Build history of the part. All positions in model axes, mm. Round coordinates to 2 decimals unless told otherwise and drop trailing zeros. Write each loop counter-clockwise with the first axis right and the second up, starting at its lowest first coordinate (ties: lowest second). Pieces come first, ordered by that corner, then holes.
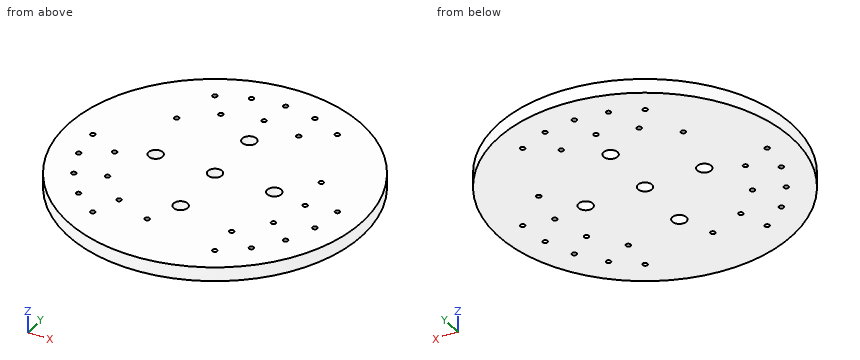
from build123d import *

# Parameters (mm, degrees)
SKETCH_R                          = 125.5
SKETCH_R_2                        = 6
PAD_DEPTH                         = 12
SKETCH001_R                       = 6
POCKET_DEPTH                      = 722.341763
POLARPATTERN_COUNT                = 4
SKETCH003_R                       = 2
POCKET001_DEPTH                   = 722.341763
SKETCH004_R                       = 2
POCKET002_DEPTH                   = 722.341763
SKETCH004_POLARPATTERN002_2_R     = 2
POCKET002_POLARPATTERN002_2_DEPTH = 722.341763
SKETCH004_POLARPATTERN002_3_R     = 2
POCKET002_POLARPATTERN002_3_DEPTH = 722.341763
SKETCH004_POLARPATTERN002_4_R     = 2
POCKET002_POLARPATTERN002_4_DEPTH = 722.341763
SKETCH004_POLARPATTERN002_5_R     = 2
POCKET002_POLARPATTERN002_5_DEPTH = 722.341763
POLARPATTERN003_COUNT             = 3
SKETCH003_POLARPATTERN004_2_R     = 2
POCKET001_POLARPATTERN004_2_DEPTH = 722.341763
SKETCH003_POLARPATTERN004_3_R     = 2
POCKET001_POLARPATTERN004_3_DEPTH = 722.341763
SKETCH003_POLARPATTERN004_4_R     = 2
POCKET001_POLARPATTERN004_4_DEPTH = 722.341763
POLARPATTERN005_COUNT             = 3


with BuildPart() as part:
    # Sketch → Pad (new body)
    with BuildSketch(Plane.XY):
        Circle(SKETCH_R)
        Circle(SKETCH_R_2, mode=Mode.SUBTRACT)
    extrude(amount=PAD_DEPTH)

    # Sketch001 → Pocket (cut, through all)
    with BuildSketch(Plane(origin=(0, 0, 0), x_dir=(-1, 0, 0), z_dir=(0, 0, -1))):
        with Locations((0, 50)):
            Circle(SKETCH001_R)
    pocket = extrude(amount=-POCKET_DEPTH, mode=Mode.SUBTRACT)

    # PolarPattern: Pocket ×4 about axis
    polarpattern_axis = Axis((0, 0, 0), (0, 0, -1))
    for i in range(1, POLARPATTERN_COUNT):
        add(pocket.rotate(polarpattern_axis, i * 360 / POLARPATTERN_COUNT), mode=Mode.SUBTRACT)

    # Sketch003 → Pocket001 (cut, through all)
    with BuildSketch(Plane.XY.offset(12)):
        with Locations((28.131884, 73.286063)):
            Circle(SKETCH003_R)
    pocket001 = extrude(amount=-POCKET001_DEPTH, mode=Mode.SUBTRACT)

    # Sketch004 → Pocket002 (cut, through all)
    with BuildSketch(Plane.XY.offset(12)):
        with Locations((51.453015, 89.227727)):
            Circle(SKETCH004_R)
    pocket002 = extrude(amount=-POCKET002_DEPTH, mode=Mode.SUBTRACT)

    # Sketch004 PolarPattern002 2 → Pocket002 PolarPattern002 2 (cut, through all)
    with BuildSketch(Plane(origin=(0, 0, 12), x_dir=(0.965789, 0.259328, 0), z_dir=(0, 0, 1))):
        with Locations((51.453015, 89.227727)):
            Circle(SKETCH004_POLARPATTERN002_2_R)
    pocket002_polarpattern002_2 = extrude(amount=-POCKET002_POLARPATTERN002_2_DEPTH, mode=Mode.SUBTRACT)

    # Sketch004 PolarPattern002 3 → Pocket002 PolarPattern002 3 (cut, through all)
    with BuildSketch(Plane(origin=(0, 0, 12), x_dir=(0.865498, 0.500912, 0), z_dir=(0, 0, 1))):
        with Locations((51.453015, 89.227727)):
            Circle(SKETCH004_POLARPATTERN002_3_R)
    pocket002_polarpattern002_3 = extrude(amount=-POCKET002_POLARPATTERN002_3_DEPTH, mode=Mode.SUBTRACT)

    # Sketch004 PolarPattern002 4 → Pocket002 PolarPattern002 4 (cut, through all)
    with BuildSketch(Plane(origin=(0, 0, 12), x_dir=(0.705989, 0.708223, 0), z_dir=(0, 0, 1))):
        with Locations((51.453015, 89.227727)):
            Circle(SKETCH004_POLARPATTERN002_4_R)
    pocket002_polarpattern002_4 = extrude(amount=-POCKET002_POLARPATTERN002_4_DEPTH, mode=Mode.SUBTRACT)

    # Sketch004 PolarPattern002 5 → Pocket002 PolarPattern002 5 (cut, through all)
    with BuildSketch(Plane(origin=(0, 0, 12), x_dir=(0.498175, 0.867077, 0), z_dir=(0, 0, 1))):
        with Locations((51.453015, 89.227727)):
            Circle(SKETCH004_POLARPATTERN002_5_R)
    pocket002_polarpattern002_5 = extrude(amount=-POCKET002_POLARPATTERN002_5_DEPTH, mode=Mode.SUBTRACT)

    # PolarPattern003: Pocket002, Pocket002 PolarPattern002 2, Pocket002 PolarPattern002 3, Pocket002 PolarPattern002 4, Pocket002 PolarPattern002 5 ×3 about axis
    polarpattern003_axis = Axis((0, 0, 12), (0, 0, 1))
    for i in range(1, POLARPATTERN003_COUNT):
        add(pocket002.rotate(polarpattern003_axis, i * 360 / POLARPATTERN003_COUNT), mode=Mode.SUBTRACT)
        add(pocket002_polarpattern002_2.rotate(polarpattern003_axis, i * 360 / POLARPATTERN003_COUNT), mode=Mode.SUBTRACT)
        add(pocket002_polarpattern002_3.rotate(polarpattern003_axis, i * 360 / POLARPATTERN003_COUNT), mode=Mode.SUBTRACT)
        add(pocket002_polarpattern002_4.rotate(polarpattern003_axis, i * 360 / POLARPATTERN003_COUNT), mode=Mode.SUBTRACT)
        add(pocket002_polarpattern002_5.rotate(polarpattern003_axis, i * 360 / POLARPATTERN003_COUNT), mode=Mode.SUBTRACT)

    # Sketch003 PolarPattern004 2 → Pocket001 PolarPattern004 2 (cut, through all)
    with BuildSketch(Plane(origin=(0, 0, 12), x_dir=(0.913545, 0.406737, 0), z_dir=(0, 0, 1))):
        with Locations((28.131884, 73.286063)):
            Circle(SKETCH003_POLARPATTERN004_2_R)
    pocket001_polarpattern004_2 = extrude(amount=-POCKET001_POLARPATTERN004_2_DEPTH, mode=Mode.SUBTRACT)

    # Sketch003 PolarPattern004 3 → Pocket001 PolarPattern004 3 (cut, through all)
    with BuildSketch(Plane(origin=(0, 0, 12), x_dir=(0.669131, 0.743145, 0), z_dir=(0, 0, 1))):
        with Locations((28.131884, 73.286063)):
            Circle(SKETCH003_POLARPATTERN004_3_R)
    pocket001_polarpattern004_3 = extrude(amount=-POCKET001_POLARPATTERN004_3_DEPTH, mode=Mode.SUBTRACT)

    # Sketch003 PolarPattern004 4 → Pocket001 PolarPattern004 4 (cut, through all)
    with BuildSketch(Plane(origin=(0, 0, 12), x_dir=(0.309017, 0.951057, 0), z_dir=(0, 0, 1))):
        with Locations((28.131884, 73.286063)):
            Circle(SKETCH003_POLARPATTERN004_4_R)
    pocket001_polarpattern004_4 = extrude(amount=-POCKET001_POLARPATTERN004_4_DEPTH, mode=Mode.SUBTRACT)

    # PolarPattern005: Pocket001, Pocket001 PolarPattern004 2, Pocket001 PolarPattern004 3, Pocket001 PolarPattern004 4 ×3 about axis
    polarpattern005_axis = Axis((0, 0, 12), (0, 0, 1))
    for i in range(1, POLARPATTERN005_COUNT):
        add(pocket001.rotate(polarpattern005_axis, i * 360 / POLARPATTERN005_COUNT), mode=Mode.SUBTRACT)
        add(pocket001_polarpattern004_2.rotate(polarpattern005_axis, i * 360 / POLARPATTERN005_COUNT), mode=Mode.SUBTRACT)
        add(pocket001_polarpattern004_3.rotate(polarpattern005_axis, i * 360 / POLARPATTERN005_COUNT), mode=Mode.SUBTRACT)
        add(pocket001_polarpattern004_4.rotate(polarpattern005_axis, i * 360 / POLARPATTERN005_COUNT), mode=Mode.SUBTRACT)


solid = part.part
1) Slice it at C-C (y = 109.5). Write the cut outline in (x, z), plus the area to 3 significant figures.
Results:
outline: (-61.32, 0) - (61.32, 0) - (61.32, 12) - (-61.32, 12) - close
area: 1,470 mm2
2) Pin check, flat tips, straight feed: pin 1 Ø3.5 at (x, y) = (-4.11, 78.39) entering from -Z; pin 2 Ø5 at (y, z) = (85, 7.5) entering from +X; pin 3 Ø2 at (x, z) = (73, 9) entering from +Y; pin 4 Ø3 at (y, z) = (-15, 5.5) entering from -X. Stop position of each tip, or through.
Results:
pin 1: passes through
pin 2: stops at x = 94.57
pin 3: stops at y = 102.79
pin 4: stops at x = -124.77
3) Wall check: L1, parallel to X at y = -74.5, z = 4.25; L2, parallel to X at y = -26, z = 4; L3, parallel to X at y = -36.5, z = 5.5. Give the ranges that are in metal, low to high.
Results:
L1: x = -101 to -73.98, -71.37 to 71.93, 73.89 to 101
L2: x = -122.78 to -101.31, -97.61 to 97.6, 101.5 to 122.78
L3: x = -120.07 to 68.14, 71.75 to 120.07
4) Slice it at B-B (y = 39). Write the cut outline in (x, z).
Results:
outline: (-119.29, 0) - (119.29, 0) - (119.29, 12) - (-119.29, 12) - close
5) Slice it at A-A (z = 3.25). Count the separate pieces of the cut face and the enclosed holes in it, plus the area to 3 significant figures.
Results:
separate pieces: 1
enclosed holes: 32
area: 48,600 mm2
